from build123d import *

# Parameters (mm, degrees)
SKETCH1_W                    = 16
SKETCH1_H                    = 48.167640012
SKETCH1_R                    = 4
BOSS_EXTRUDE1_DEPTH          = 3.175
EDGE_FLANGE1_STRIP_W         = 19.05
EDGE_FLANGE1_STRIP_H         = 3.175
EDGE_FLANGE1_STRIP_CUT_DEPTH = 16
EDGE_FLANGE1_DEPTH           = 16
EDGE_FLANGE1_START           = 3.175
EDGE_FLANGE1_FLAT_DEPTH      = 3.175
SKETCH11_R                   = 3.7210804
CUT_EXTRUDE1_DEPTH           = 81.232501141
M8_CLEARANCE_HOLE1_D         = 9
FILLET1_R                    = 2.54


# Sheet-metal steps are written as plain solids
with BuildPart() as part:
    # Sketch1 → Boss-Extrude1 (new body)
    with BuildSketch(Plane(origin=(0, 0, 0), x_dir=(1, 0, 0), z_dir=(0, 1, 0))):
        with Locations((0, 16.083820006)):
            Rectangle(SKETCH1_W, SKETCH1_H)
        with Locations(Location((0, 0, 0), (0, 0, 270))):
            Circle(SKETCH1_R, mode=Mode.SUBTRACT)
    extrude(amount=BOSS_EXTRUDE1_DEPTH)

    # Edge-Flange1 strip (across the edge) → Edge-Flange1 strip cut (cut)
    with BuildSketch(Plane(origin=(8, 3.175, -40.167640012), x_dir=(0, 0, 1), z_dir=(-1, 0, 0))):
        with Locations((-6.35, -1.5875)):
            Rectangle(EDGE_FLANGE1_STRIP_W, EDGE_FLANGE1_STRIP_H)
    extrude(amount=EDGE_FLANGE1_STRIP_CUT_DEPTH, mode=Mode.SUBTRACT)

    # Edge-Flange1 bend section (across the edge) → Edge-Flange1 (add)
    with BuildSketch(Plane(origin=(8, 3.175, -40.167640012), x_dir=(0, 0, 1), z_dir=(-1, 0, 0))):
        with BuildLine():
            Line((-3.175, 3.175), (0, 3.175))
            ThreePointArc((0, 3.175), (0.92993597, 0.92993597), (3.175, 0))
            Line((3.175, 0), (3.175, -3.175))
            ThreePointArc((3.175, -3.175), (-1.315128061, -1.315128061), (-3.175, 3.175))
        make_face()
    extrude(amount=EDGE_FLANGE1_DEPTH)

    # Edge-Flange1 profile (on flange) → Edge-Flange1 flat (add)
    with BuildSketch(Plane(origin=(0, 3.175, -40.167640012), x_dir=(-1, 0, 0), z_dir=(0, 0, -1)).offset(EDGE_FLANGE1_START)):
        Polygon((8, 3.175), (8, 47.359), (-8, 47.359), (-27.7, 47.359), (-35.32, 47.359), (-35.32, 29.325), (-27.7, 29.325), (-8, 29.325), (-8, 3.175), align=None)
    extrude(amount=-EDGE_FLANGE1_FLAT_DEPTH)

    # Sketch11 → Cut-Extrude1 (cut, through all)
    with BuildSketch(Plane(origin=(0, 0, -43.342640012), x_dir=(-1, 0, 0), z_dir=(0, 0, -1))):
        with Locations(Location((-24.4742, 41.517, 0), (0, 0, 90))):
            Circle(SKETCH11_R)
    extrude(amount=-CUT_EXTRUDE1_DEPTH, mode=Mode.SUBTRACT)

    # M8 Clearance Hole1 (through all)
    with Locations(Plane(origin=(0, 0, -43.342640012), x_dir=(-1, 0, 0), z_dir=(0, 0, -1))):
        with Locations((-24.4742, 41.517)):
            Hole(M8_CLEARANCE_HOLE1_D / 2)

    # Fillet1
    fillet1_edges = [part.edges().sort_by_distance(p)[0] for p in [
        (8, 32.5, -41.755140012),
        (-8, 50.534, -41.755140012),
        (35.32, 50.534, -41.755140012),
        (35.32, 32.5, -41.755140012),
        (8, 1.5875, 8),
        (-8, 1.5875, 8),
    ]]
    fillet(fillet1_edges, radius=FILLET1_R)


solid = part.part
Check sheet for the modelled part. Datum: model origin and axes. Units: mm. A direction names the side the tool comes from. Give positions to 0.01 mm unless a question says otherwise; leave off trailing zeros. Write each loop counter-clockwise with the first axis right and the second up, starting at its lowest first coordinate (ties: lowest second). Pieces come first, ordered by that corner, then holes. Notation, with made-up numbers: (51, 32) -> (110, 32) arc R23 cw to (110, 56) -> close; hole circle Ø6 at (77, 36.25). An arc over 180 degrees is marked (long way). Use one line per item in the form item = value. Start each with the question number.
1. Mould release check, pull along Z, two halves, no side actions. Record for faces 1 (the cylindrical face through (-3.905, 1.565, -0.867)), 2 (the flat face through (35.32, 42, -42)), 3 (the flat face through (0, 2, 8)): pulls with the +Z half, pulls with the -Z half, needs draft (parallel to the pull), parting line crosses it, or undercut.
2. Section check C-C (y = 43). Record the cut outline in (x, z), and give its area (3 significant figures).
3. Section check D-D (x = 17). Record the cut outline in (y, z), and give its area (3 significant figures).
4. Section check A-A (z = 0). Record the cut outline in (x, y) (3 decimals).
5. Section check B-B (x = 0). Record the cut outline in (y, z) (3 decimals), and give its area (3 significant figures).
6. Access from +Z, -Z, +X, -X, +Y, -Y to the whole of each face (thin tool, end or side, straight path). Record for faces 4 (the cylindrical face through (34.556, 49.81, -41.733)), 5 (the flat face through (8, 3, -26)), 6 (the flat face through (9, 34, -40.168)).
7. Thickness scan on line 1 along Y through (x, z) = (0, -20) (3 decimals); line 2 along Z through (x, y) = (-5, 19.5). Record the ranges inside material, lowest first. Write a range as from..to.
8. Go/stop test with flat-tipped pins: P1, Ø1.5, axis at x = 16.5, y = 43, coming from the +Z side; P2, Ø5.5, axis at x = 24.47, y = 41.52, coming from the -Z side; P3, Ø9, axis at x = 0, z = 0, coming from the -Y side; P4, Ø17.5, axis at x = 0.5, z = -21.5, coming from the +Y side (3 decimals). Record where each tip stops, or that it passes through.
Conclusion:
q1.face_1 = undercut
q1.face_2 = needs draft
q1.face_3 = pulls with the +Z half
q2.outline = (-8, -43.34) -> (20.23, -43.34) -> (20.23, -40.17) -> (-8, -40.17) -> close; (28.72, -43.34) -> (35.32, -43.34) -> (35.32, -40.17) -> (28.72, -40.17) -> close
q2.area = 111 mm²
q3.outline = (32.5, -43.34) -> (50.53, -43.34) -> (50.53, -40.17) -> (32.5, -40.17) -> close
q3.area = 57.3 mm²
q4.outline = (-8, 0) -> (-4, 0) -> (-4, 3.175) -> (-8, 3.175) -> close; (4, 0) -> (8, 0) -> (8, 3.175) -> (4, 3.175) -> close
q5.outline = (0, -36.993) arc R6.35 ccw to (6.35, -43.343) -> (50.534, -43.343) -> (50.534, -40.168) -> (6.35, -40.168) arc R3.175 cw to (3.175, -36.993) -> (3.175, -4) -> (0, -4) -> close; (0, 4) -> (3.175, 4) -> (3.175, 8) -> (0, 8) -> close
q5.area = 281 mm²
q6.face_4 = +Z, -Z, +X, +Y
q6.face_5 = +Z, -Z, +X, -Y
q6.face_6 = +Z, +X, -X, +Y
q7.line_1 = 0..3.175
q7.line_2 = -43.34..-40.17
q8.P1 = -40.17
q8.P2 = through
q8.P3 = 0
q8.P4 = 3.175
